Source: three-view drawing plus pictorial views. Frame: mm from the lowest corner of the part. Round coordinates to 2 decimals unless told otherwise and drop trailing zeros. Loops run counter-clockwise (first coordinate to the right, second up) from the corner with the lowest first, then second, coordinate; pieces in that order, holes last. Notation, with made-up numbers: (7, 0.25) -> (40, 0.25) arc R10 cw to (40, 14.25) -> close; hole circle Ø8 at (-6, -2.5). An arc over 180 degrees is marked (long way). Answer in a Markdown table with one row per item. Add a question column.
Q1. Section C-C, the plane z = 73.5. Output: boundary loops of the cut face in (x, y).
Q2. Section A-A, the plane y = 120. Output: boundary loops of the cut face in (x, z).
Q3. Pin query (flat end, axial travel): pin 1 (25 mm diameter, centred on y = 33.5, z = 86, fed in from -X); pin 2 (25 mm diameter, centred on x = 18, y = 138, fed in from +Z). Return the tip coordinate at first contact, or that it passes through.
Q4. Section B-B, the plane x = 96.5. Output: boundary loops of the cut face in (y, z), and give its area (3 significant figures).
Q5. Ray query, L1, parallel to Y at x = 388.5, z = 17.5; L2, parallel to X at y = 34, z = 80; L3, parallel to Z at x = 312.5, y = 381.5. Return the intervals inside material, ascending. Write a range as from..to.
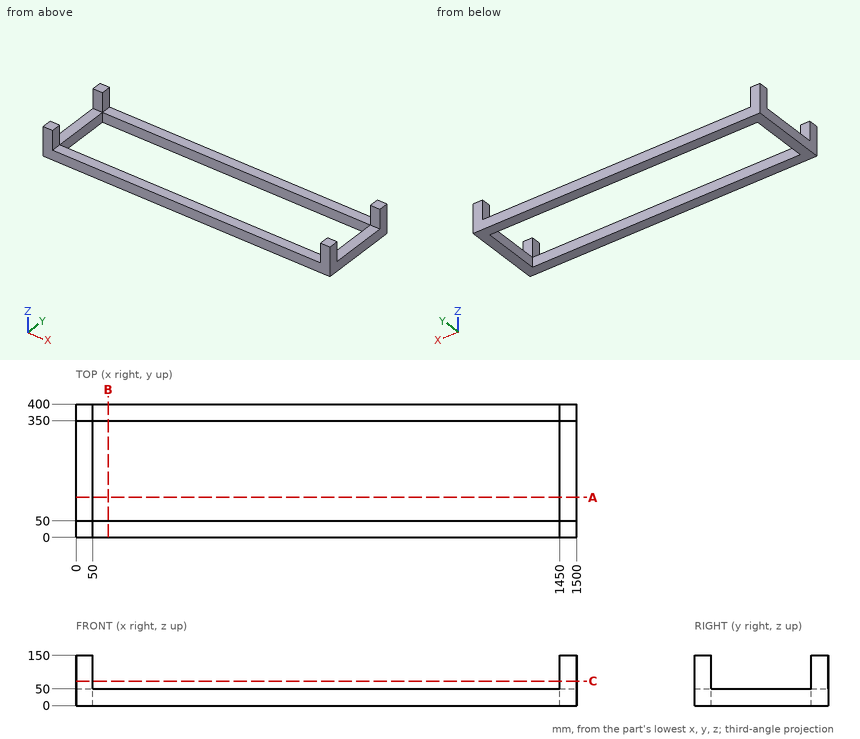
Answer block:
| question | item | result |
|---|---|---|
| 1 | outline | (0, 0) -> (50, 0) -> (50, 50) -> (0, 50) -> close; (0, 350) -> (50, 350) -> (50, 400) -> (0, 400) -> close; (1450, 0) -> (1500, 0) -> (1500, 50) -> (1450, 50) -> close; (1450, 350) -> (1500, 350) -> (1500, 400) -> (1450, 400) -> close |
| 2 | outline | (0, 0) -> (50, 0) -> (50, 50) -> (0, 50) -> close; (1450, 0) -> (1500, 0) -> (1500, 50) -> (1450, 50) -> close |
| 3 | pin 1 | x = 0 |
| 3 | pin 2 | z = 50 |
| 4 | outline | (0, 0) -> (50, 0) -> (50, 50) -> (0, 50) -> close; (350, 0) -> (400, 0) -> (400, 50) -> (350, 50) -> close |
| 4 | area | 5,000 mm^2 |
| 5 | L1 | 0..50, 350..400 |
| 5 | L2 | 0..50, 1450..1500 |
| 5 | L3 | 0..50 |
